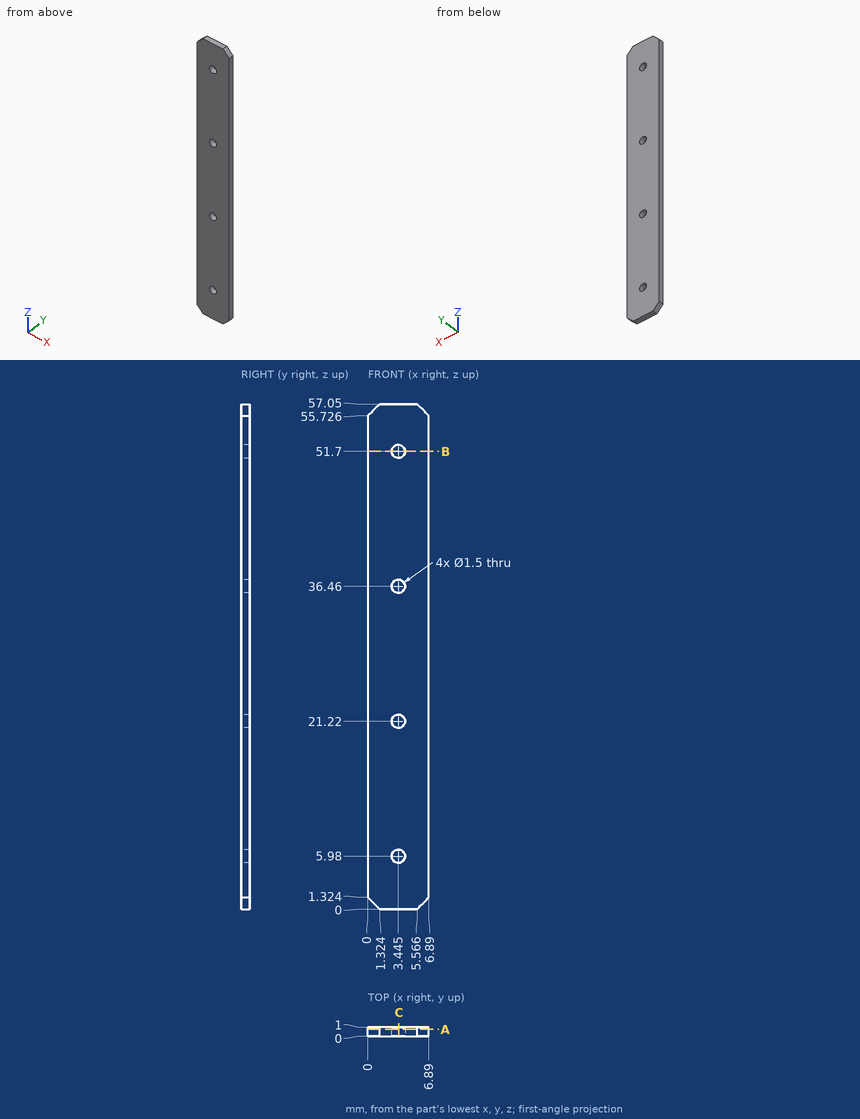
Answer from the drawing. Dimensions are ordinates in mm from the lowest x, y and z of the part. Coordinates: 2 decimals unless noted, no trailing zeros. Write each loop counter-clockwise with the first axis right and the second up, starting at its lowest first coordinate (ties: lowest second). Pieces come first, ordered by that corner, then holes. Notation, with made-up numbers: (78, -33.5) - (116, -33.5) arc R15 ccw to (116, -9.5) - close; hole circle Ø3 at (38, 47.5). An arc over 180 degrees is marked (long way). Return JSON: item names as keys, results as strings. Group by question number.
Q1. The part is cut by section A-A on y = 0.75. State how many separate pieces and enclosed holes the cut face has.
Q2. The part is cut by section C-C on x = 3.5. Write down the section's boundary in (y, z).
Q3. The part is cut by section B-B on z = 51.7. Write down the section's boundary in (x, y) (3 decimals).
Q4. Find the intervals of material crossed by line 1 along X through (y, z) = (0.35, 36.46) (3 decimals); line 2 along Z through (x, y) = (3, 0.1); line 3 along Z through (x, y) = (0.75, 0.5) (1 decimal), in increasing order. Write a range as [from, to].
Evaluation:
{
 "1": {"separate pieces": "1", "enclosed holes": "4"},
 "2": {"outline": "(0, 0) - (1, 0) - (1, 5.23) - (0, 5.23) - close; (0, 6.73) - (1, 6.73) - (1, 20.47) - (0, 20.47) - close; (0, 21.97) - (1, 21.97) - (1, 35.71) - (0, 35.71) - close; (0, 37.21) - (1, 37.21) - (1, 50.95) - (0, 50.95) - close; (0, 52.45) - (1, 52.45) - (1, 57.05) - (0, 57.05) - close"},
 "3": {"outline": "(0, 0) - (2.695, 0) - (2.695, 1) - (0, 1) - close; (4.195, 0) - (6.89, 0) - (6.89, 1) - (4.195, 1) - close"},
 "4": {"line 1": "x = [0, 2.695], [4.195, 6.89]", "line 2": "z = [0, 5.38], [6.58, 20.62], [21.82, 35.86], [37.06, 51.1], [52.3, 57.05]", "line 3": "z = [0.6, 56.5]"}
}
